For this review, use the dimensioned drawing (mm, ordinates from the lowest corner) and the shaded views. Coordinates: 2 decimals unless noted, no trailing zeros. Order: outer loops, then holes, each group sorted by start corner. A loop starts at its lowest first (then second) coordinate and runs counter-clockwise, first axis right, second up. Notation, with made-up numbers: (-4.75, -1.5) -> (0.25, -1.5) arc R26 cw to (0.25, 30.5) -> close; hole circle Ø2 at (-30, 80). An arc over 180 degrees is marked (long way). Use one line per item in the form item = value. Start each with the question number.
(1) Take a section at D-D (z = 30.5). State the section outline as (x, y) points.
(2) Take a section at B-B (x = 11.25). State the section outline as (y, z) points.
(3) Take a section at C-C (y = 0.7). State how many separate pieces and enclosed holes the cut face has.
(4) Take a section at A-A (x = 3.75). State the section outline as (y, z) points (1 decimal).
(5) Wall thickness on line 1 along X through (y, z) = (0.75, 51); line 2 along X through (y, z) = (0.3, 60.5) (1 decimal); line 3 along X through (y, z) = (2, 4) (1 decimal): over which ranges is each line inside the solid? List them lowest first.
(6) Insertion check: pin 1 Ø1.5 at (x, y) = (9.5, 0.5) entering from -Z; pin 2 Ø3.5 at (x, z) = (3.18, 27.04) entering from +Y; pin 3 Ø1.5 at (y, z) = (2, 41.5) entering from +X. Each pin has a flat end and moves straight along its axis. Give the tip position at first contact, or say it passes through.
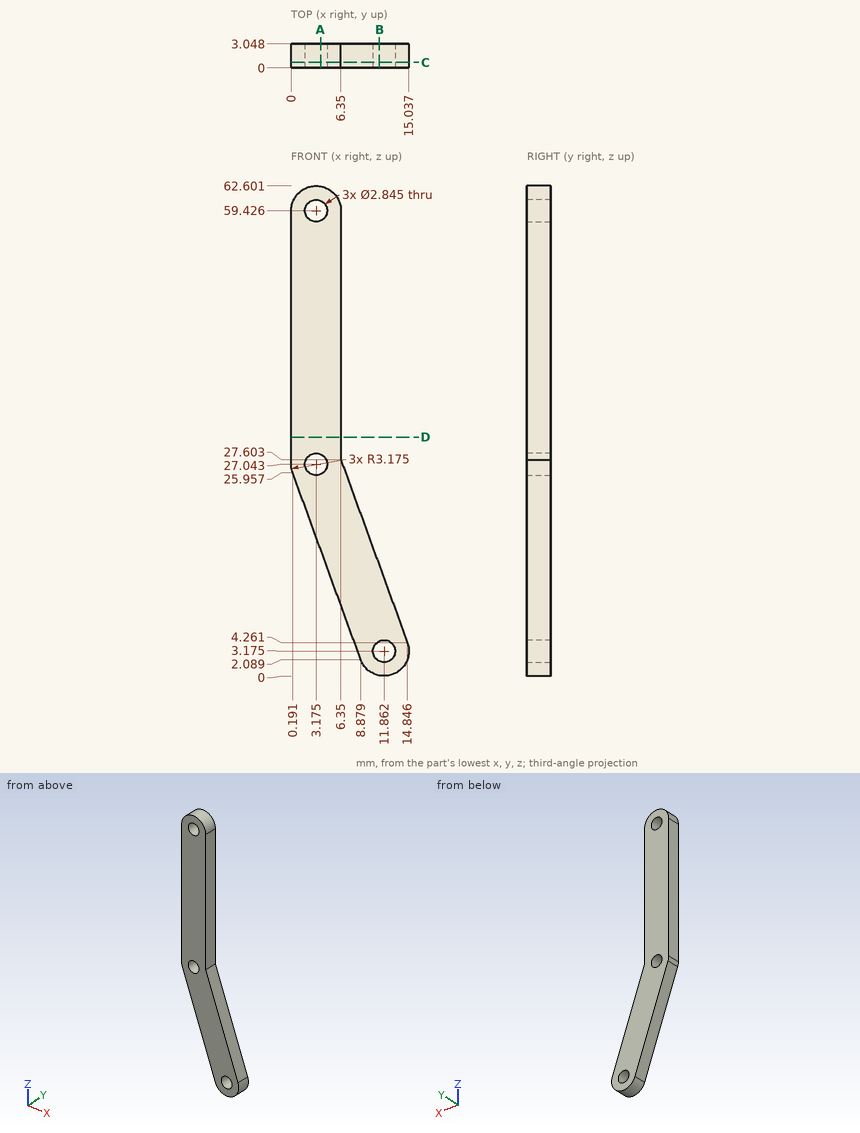
Findings:
q1.outline = (0, 0) -> (6.35, 0) -> (6.35, 3.05) -> (0, 3.05) -> close
q2.outline = (0, 0.06) -> (3.05, 0.06) -> (3.05, 1.89) -> (0, 1.89) -> close; (0, 4.46) -> (3.05, 4.46) -> (3.05, 14.14) -> (0, 14.14) -> close
q3.separate_pieces = 1
q3.enclosed_holes = 3
q4.outline = (0, 16.2) -> (3, 16.2) -> (3, 25.7) -> (0, 25.7) -> close; (0, 28.3) -> (3, 28.3) -> (3, 58.1) -> (0, 58.1) -> close; (0, 60.7) -> (3, 60.7) -> (3, 62.5) -> (0, 62.5) -> close
q5.line_1 = 0 to 6.35
q5.line_2 = 0.2 to 2.2, 4.1 to 6.2
q5.line_3 = 8.2 to 10.7, 13 to 14.9
q6.pin_1 = 0.44
q6.pin_2 = 3.05
q6.pin_3 = 6.35
